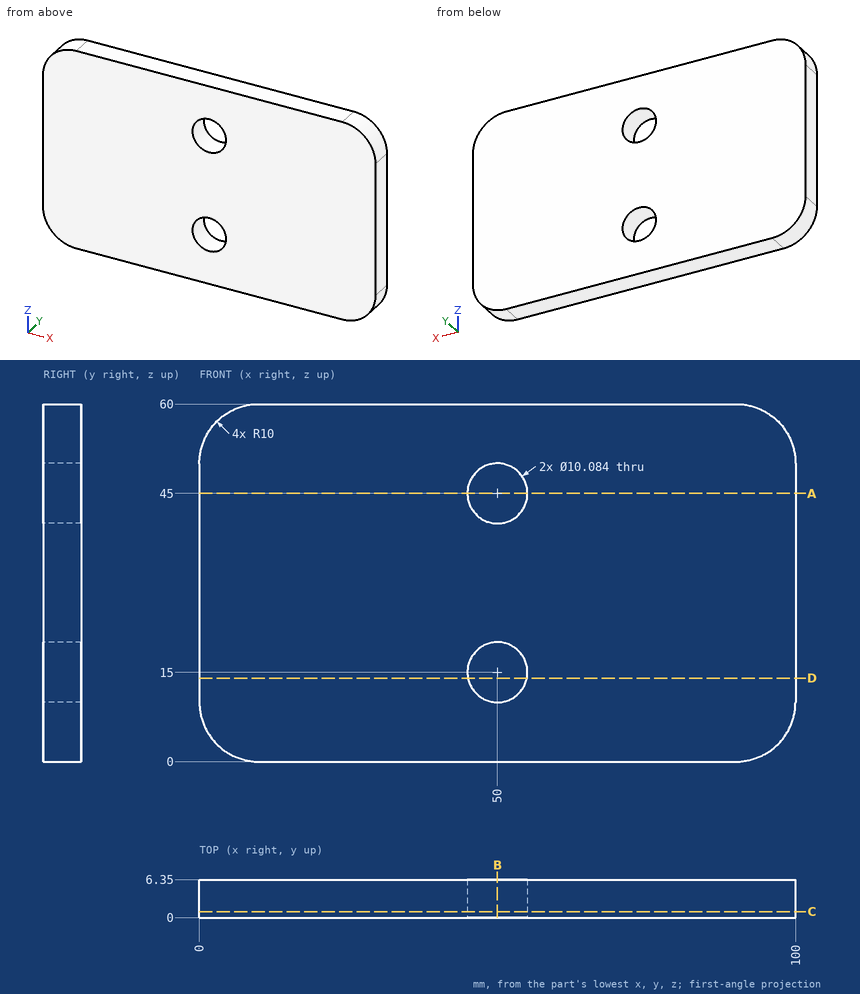
Geometry: see drawing. Coordinates: mm, zero at the bounding-box minimum. Coordinates: 2 decimals unless noted, no trailing zeros. Loops run counter-clockwise (first coordinate to the right, second up) from the corner with the lowest first, then second, coordinate; pieces in that order, holes last. Notation, with made-up numbers: (57, 34.5) - (112, 34.5) arc R27 cw to (112, 67.5) - close; hole circle Ø9 at (-35.75, 49). An arc over 180 degrees is marked (long way). Answer in a Markdown table with one row per item.
(1) Cut plane A-A on z = 45. Output: boundary loops of the cut face in (x, y), plus the area to 3 significant figures.
Model answer:
| item | result |
|---|---|
| outline | (0, 0) - (44.96, 0) - (44.96, 6.35) - (0, 6.35) - close; (55.04, 0) - (100, 0) - (100, 6.35) - (55.04, 6.35) - close |
| area | 571 mm² |
(2) Cut plane B-B on x = 50. Output: boundary loops of the cut face in (y, z).
Model answer:
| item | result |
|---|---|
| outline | (0, 0) - (6.35, 0) - (6.35, 9.96) - (0, 9.96) - close; (0, 20.04) - (6.35, 20.04) - (6.35, 39.96) - (0, 39.96) - close; (0, 50.04) - (6.35, 50.04) - (6.35, 60) - (0, 60) - close |
(3) Material intervals for L1, parallel to Z at x = 50, y = 4.5; L2, parallel to X at y = 1, z = 15.5; L3, parallel to X at y = 4.5, z = 16.5, sorted ascending. Write a range as from..to.
Model answer:
| item | result |
|---|---|
| L1 | z = 0..9.96, 20.04..39.96, 50.04..60 |
| L2 | x = 0..44.98, 55.02..100 |
| L3 | x = 0..45.19, 54.81..100 |
(4) Cut plane C-C on y = 1. Output: boundary loops of the cut face in (x, z), plus the area to 3 significant figures.
Model answer:
| item | result |
|---|---|
| outline | (0, 10) arc R10 ccw to (10, 0) - (90, 0) arc R10 ccw to (100, 10) - (100, 50) arc R10 ccw to (90, 60) - (10, 60) arc R10 ccw to (0, 50) - close; hole circle Ø10.08 at (50, 15); hole circle Ø10.08 at (50, 45) |
| area | 5,750 mm² |
(5) Cut plane D-D on z = 14. Output: boundary loops of the cut face in (x, y), plus the area to 3 significant figures.
Model answer:
| item | result |
|---|---|
| outline | (0, 0) - (45.06, 0) - (45.06, 6.35) - (0, 6.35) - close; (54.94, 0) - (100, 0) - (100, 6.35) - (54.94, 6.35) - close |
| area | 572 mm² |
